Here's how the part is built. I have some questions about the finished solid (model axes, mm). A direction names the side the tool comes from. Round coordinates to 2 decimals unless told otherwise and drop trailing zeros. Loops run counter-clockwise (first coordinate to the right, second up) from the corner with the lowest first, then second, coordinate; pieces in that order, holes last. Notation, with made-up numbers: M 7.5,19 L 58.5,19 A19 ccw 58.5,30 Z; hole C -14,-1.75 d4. An arc over 180 degrees is marked long. Use a Markdown table: item, result.
from build123d import *

# Parameters (mm, degrees)
ESQUISSE1_R                           = 4.05
T_LE_DE_BASE_PLI_E1_DEPTH             = 2.5
T_LE_PLI_E_SUR_AR_TE1_STRIP_W         = 11.4732
T_LE_PLI_E_SUR_AR_TE1_STRIP_H         = 2.5
T_LE_PLI_E_SUR_AR_TE1_STRIP_CUT_DEPTH = 130
T_LE_PLI_E_SUR_AR_TE1_DEPTH           = 130
CONG_1_R                              = 3
ENL_V_MAT_EXTRU_1_DEPTH               = 10


# Sheet-metal steps are written as plain solids
with BuildPart() as part:
    # Esquisse1 → Tôle de base pliée1 (new body)
    with BuildSketch(Plane.XY):
        with BuildLine():
            Line((0, 0), (130, 0))
            Line((130, 0), (130, 22))
            ThreePointArc((130, 22), (65, 87), (0, 22))
            Line((0, 22), (0, 0))
        make_face()
        with Locations((65, 22)):
            Circle(ESQUISSE1_R, mode=Mode.SUBTRACT)
        with BuildLine():
            ThreePointArc((123.2, 22), (65, 80.2), (6.8, 22))
            ThreePointArc((6.8, 22), (10.9, 17.9), (15, 22))
            ThreePointArc((15, 22), (65, 72), (115, 22))
            ThreePointArc((115, 22), (119.1, 17.9), (123.2, 22))
        make_face(mode=Mode.SUBTRACT)
    extrude(amount=-T_LE_DE_BASE_PLI_E1_DEPTH)

    # Tôle pliée sur arête1 strip (across the edge) → Tôle pliée sur arête1 strip cut (cut)
    with BuildSketch(Plane.YZ):
        with Locations((-2.5, -1.25)):
            Rectangle(T_LE_PLI_E_SUR_AR_TE1_STRIP_W, T_LE_PLI_E_SUR_AR_TE1_STRIP_H)
    extrude(amount=T_LE_PLI_E_SUR_AR_TE1_STRIP_CUT_DEPTH, mode=Mode.SUBTRACT)

    # Tôle pliée sur arête1 section (across the edge) → Tôle pliée sur arête1 (add)
    with BuildSketch(Plane.YZ):
        with BuildLine():
            Line((0, 0.7366), (0, 27.5))
            Line((0, 27.5), (2.5, 27.5))
            Line((2.5, 27.5), (2.5, 0.7366))
            ThreePointArc((2.5, 0.7366), (2.715745145, 0.215745145), (3.2366, 0))
            Line((3.2366, 0), (3.2366, -2.5))
            ThreePointArc((3.2366, -2.5), (0.947978192, -1.552021808), (0, 0.7366))
        make_face()
    extrude(amount=T_LE_PLI_E_SUR_AR_TE1_DEPTH)

    # Congé1
    cong_1_edges = [part.edges().sort_by_distance(p)[0] for p in [
        (0, 1.25, 27.5),
        (130, 1.25, 27.5),
    ]]
    fillet(cong_1_edges, radius=CONG_1_R)

    # Esquisse9 → Enlèv. mat.-Extru.1 (cut)
    with BuildSketch(Plane(origin=(0, 2.5, 0), x_dir=(1, 0, 0), z_dir=(0, 1, 0))):
        with BuildLine():
            Line((18.15, -13.25), (18.15, -20.65))
            ThreePointArc((18.15, -20.65), (15, -23.8), (11.85, -20.65))
            Line((11.85, -20.65), (11.85, -13.25))
            ThreePointArc((11.85, -13.25), (15, -10.1), (18.15, -13.25))
        make_face()
        with BuildLine():
            Line((111.85, -13.25), (111.85, -20.65))
            ThreePointArc((111.85, -20.65), (115, -23.8), (118.15, -20.65))
            Line((118.15, -20.65), (118.15, -13.25))
            ThreePointArc((118.15, -13.25), (115, -10.1), (111.85, -13.25))
        make_face()
    extrude(amount=-ENL_V_MAT_EXTRU_1_DEPTH, mode=Mode.SUBTRACT)


solid = part.part
1. We'd pull the mould along Y, two halves only. Please class faces 6 (the face through (64.09, 0.973, -1.577)), 7 (the face through (14.9, 1.3, 10.1)), 8 (the face through (119, 17.9, -1.2)): +Y half, -Y half, draft (parallel to the pull), parting line (faces both ways), or undercut.
Answer sheet:
| item | result |
|---|---|
| face 6 | -Y half |
| face 7 | draft |
| face 8 | undercut |
2. Which directions (+Z, -Z, +X, -X, +Y, -Y) give clear straight access to the entire face, cutting with the end or side of a thin tool? Please do faces 1 (the face through (64, 1, 27.5)), 2 (the face through (118.15, 1, 17)), 3 (the face through (129.1, 1.27, 26.64)), 4 (the face through (64, 2.5, 14)), 5 (the face through (10.8, 17.9, -1.2)).
Answer sheet:
| item | result |
|---|---|
| face 1 | +Z, +X, -X, +Y, -Y |
| face 2 | +Y, -Y |
| face 3 | +Z, +X, +Y, -Y |
| face 4 | +Z, +X, -X, +Y |
| face 5 | +Z, -Z |
3. Imagine slicing it at C-C, the plane y = 59.5. Write out the boundary of the cut face in (x, z).
Answer sheet:
| item | result |
|---|---|
| outline | M 11.91,-2.5 L 20.49,-2.5 L 20.49,0 L 11.91,0 Z; M 31.93,-2.5 L 98.07,-2.5 L 98.07,0 L 31.93,0 Z; M 109.51,-2.5 L 118.09,-2.5 L 118.09,0 L 109.51,0 Z |
4. For pin 1 Ø2 at (x, z) = (38, 15.5) entering from +Y; pin 2 Ø6.5 at (x, y) = (65, 22) entering from -Z; pin 3 Ø5 at (x, y) = (53, 19) entering from +Z; pin 4 Ø6 at (y, z) = (47.5, 2) entering from -X, each with a flat end and sliding along its axis, tell me the tip position at first contact or that it passes through.
Answer sheet:
| item | result |
|---|---|
| pin 1 | y = 2.5 |
| pin 2 | through |
| pin 3 | z = 0 |
| pin 4 | x = 4.31 |
5. Imagine slicing it at A-A, the plane x = 65. Write out the boundary of the cut face in (y, z), then the cut area to 3 significant figures.
Answer sheet:
| item | result |
|---|---|
| outline | M 0,0.74 A3.24 ccw 3.24,-2.5 L 17.95,-2.5 L 17.95,0 L 3.24,0 A0.74 cw 2.5,0.74 L 2.5,27.5 L 0,27.5 Z; M 26.05,-2.5 L 72,-2.5 L 72,0 L 26.05,0 Z; M 80.2,-2.5 L 87,-2.5 L 87,0 L 80.2,0 Z |
| area | 243 mm2 |
6. Imagine slicing it at B-B, the plane z = 15.25. Write out the boundary of the cut face in (x, y).
Answer sheet:
| item | result |
|---|---|
| outline | M 0,0 L 11.85,0 L 11.85,2.5 L 0,2.5 Z; M 18.15,0 L 111.85,0 L 111.85,2.5 L 18.15,2.5 Z; M 118.15,0 L 130,0 L 130,2.5 L 118.15,2.5 Z |
7. I need wall thicknesses on probe 1 along Z at (x, y) = (51, 40); probe 2 along Y at (x, z) = (99.5, 21.5); probe 3 along X at (y, z) = (46.5, -0.25). Which ranges of each line are inside material? Lowest first, please. Write a range as from..to.
Answer sheet:
| item | result |
|---|---|
| probe 1 | -2.5..0 |
| probe 2 | 0..2.5 |
| probe 3 | 4.79..12.21, 21.41..108.59, 117.79..125.21 |
8. Imagine slicing it at D-D, the plane x = 51. Write out the boundary of the cut face in (y, z).
Answer sheet:
| item | result |
|---|---|
| outline | M 0,0.74 A3.24 ccw 3.24,-2.5 L 70,-2.5 L 70,0 L 3.24,0 A0.74 cw 2.5,0.74 L 2.5,27.5 L 0,27.5 Z; M 78.49,-2.5 L 85.47,-2.5 L 85.47,0 L 78.49,0 Z |
